Work out the finished part from the listing and answer in its coordinate system (mm). A direction names the side the tool comes from. Give positions to 0.01 mm unless a question says otherwise; leave off trailing zeros. Order: outer loops, then holes, each group sorted by start corner. A loop starts at its lowest first (then second) coordinate and runs counter-clockwise, first axis right, second up. Notation, with made-up numbers: (-11.75, 47) - (1.25, 47) arc R26 cw to (1.25, 82) - close; hole circle Ø2 at (-36.5, 75.5). An arc over 180 degrees is marked (long way). Put each result on its own line as item: value.
```python
from build123d import *

# Parameters (mm, degrees)
SKETCH1_R           = 47.6885
BOSS_EXTRUDE1_DEPTH = 3.175
SKETCH2_R           = 49.5046
BOSS_EXTRUDE2_DEPTH = 3.175
SKETCH3_R           = 3.175
SKETCH3_R_2         = 9.525
CUT_EXTRUDE1_DEPTH  = 7.35


with BuildPart() as part:
    # Sketch1 → Boss-Extrude1 (new body)
    with BuildSketch(Plane(origin=(0, 0, 0), x_dir=(1, 0, 0), z_dir=(0, 1, 0))):
        Circle(SKETCH1_R)
    extrude(amount=BOSS_EXTRUDE1_DEPTH)

    # Sketch2 → Boss-Extrude2 (add)
    with BuildSketch(Plane(origin=(0, 3.175, 0), x_dir=(1, 0, 0), z_dir=(0, 1, 0))):
        Circle(SKETCH2_R)
    extrude(amount=BOSS_EXTRUDE2_DEPTH)

    # Sketch3 → Cut-Extrude1 (cut, through all)
    with BuildSketch(Plane(origin=(0, 6.35, 0), x_dir=(1, 0, 0), z_dir=(0, 1, 0))):
        with Locations((-31.75, 0)):
            Circle(SKETCH3_R)
        with Locations((31.75, 0)):
            Circle(SKETCH3_R)
        Circle(SKETCH3_R_2)
    extrude(amount=-CUT_EXTRUDE1_DEPTH, mode=Mode.SUBTRACT)


solid = part.part
```
(1) Determine the mould class of faces 3 (the face through (-1, 6.35, 10)), 4 (the face through (-6.445, 4.74, -49.083)), 5 (the face through (-7.559, 3.219, 5.796)) for opening direction Z: pulls with the +Z half, pulls with the -Z half, needs draft (parallel to the pull), parting line crosses it, or undercut.
Geometry check:
face 3: needs draft
face 4: parting line crosses it
face 5: undercut
(2) Section A-A, the plane z = 0 is taken. Count the separate pieces of the cut face and the enclosed holes in it, then the cut area to 3 significant figures.
Geometry check:
separate pieces: 4
enclosed holes: 0
area: 416 mm²
(3) Section C-C, the plane y = 4.5 is taken. Write down the section's boundary in (x, z) (3 decimals), then the cut area to 3 significant figures.
Geometry check:
outline: circle Ø99.009 at (0, 0); hole circle Ø6.35 at (-31.75, 0); hole circle Ø19.05 at (0, 0); hole circle Ø6.35 at (31.75, 0)
area: 7,350 mm²
(4) A tool of negligible diameter and unlimited length cuts with its end or side. For faces 1 (the face through (45.486, 1.565, -14.324)), 2 (the face through (-1, 0, 10)), from which of +Z, -Z, +X, -X, +Y, -Y can it reach the whole face along a straight path? Write none if from no direction.
Geometry check:
face 1: -Y
face 2: +Z, -Z, +X, -X, -Y
(5) Section D-D, the plane z = -36 is taken. Write down the section's boundary in (x, y) (3 decimals), then the cut area to 3 significant figures.
Geometry check:
outline: (-33.981, 3.175) - (-31.276, 3.175) - (-31.276, 0) - (31.276, 0) - (31.276, 3.175) - (33.981, 3.175) - (33.981, 6.35) - (-33.981, 6.35) - close
area: 414 mm²
(6) Straight lines are drawn through the part: line 1 (X direction, y = 3.75, z = 0) (3 decimals); line 2 (X direction, y = 3, z = 0) (1 decimal); line 3 (X direction, y = 5, z = -4). For each, find the intervals that lie inside material, in ascending order.
Geometry check:
line 1: x = -49.505 to -34.925, -28.575 to -9.525, 9.525 to 28.575, 34.925 to 49.505
line 2: x = -47.7 to -34.9, -28.6 to -9.5, 9.5 to 28.6, 34.9 to 47.7
line 3: x = -49.34 to -8.64, 8.64 to 49.34
(7) Given pin 1 (1.5 mm diameter, centred on x = -31.5, y = 1.5, fed in from -Z); pin 2 (1 mm diameter, centred on x = -11.5, y = 2, fed in from +Z); pin 3 (1.5 mm diameter, centred on y = 5.5, z = -16.5, fed in from +X), each flat-ended and moving along its own axis, determine where each tip first touches the part or whether it passes through.
Geometry check:
pin 1: stops at z = -36.45
pin 2: stops at z = 46.4
pin 3: stops at x = 46.93
